from build123d import *

# Parameters (mm, degrees)
F0_R     = 42.5
F0_W     = 12
F0_H     = 12
F1_DEPTH = 15
F2_R     = 42.5
F3_DEPTH = 5
F4_R     = 2.1
F5_DEPTH = 10
F7_DEPTH = 4


with BuildPart() as f1:
    # F0 (on Top) → F1 (new body)
    with BuildSketch(Plane.XY):
        Circle(F0_R)
        Rectangle(F0_W, F0_H, mode=Mode.SUBTRACT)
    extrude(amount=F1_DEPTH)

    # F2 (on face) → F3 (join)
    with BuildSketch(Plane(origin=(0, 0, 0), x_dir=(1, 0, 0), z_dir=(0, 0, -1))):
        Circle(F2_R)
    extrude(amount=F3_DEPTH)

    # F4 (on face) → F5 (cut)
    with BuildSketch(Plane.XY.offset(15)):
        with Locations((-21.25, 0)):
            Circle(F4_R)
        with Locations((0, 21.25)):
            Circle(F4_R)
        with Locations((21.25, 0)):
            Circle(F4_R)
        with Locations((0, -21.25)):
            Circle(F4_R)
    extrude(amount=-F5_DEPTH, mode=Mode.SUBTRACT)

    # F6 (on face) → F7 (cut)
    with BuildSketch(Plane.XY.offset(15)):
        Polygon((-24.714102, 2), (-24.714102, -2), (-21.25, -4), (-17.785898, -2), (-17.785898, 2), (-21.25, 4), align=None)
        Polygon((-3.464102, 23.25), (-3.464102, 19.25), (0, 17.25), (3.464102, 19.25), (3.464102, 23.25), (0, 25.25), align=None)
        Polygon((17.785898, 2), (17.785898, -2), (21.25, -4), (24.714102, -2), (24.714102, 2), (21.25, 4), align=None)
        Polygon((-3.464102, -19.25), (-3.464102, -23.25), (0, -25.25), (3.464102, -23.25), (3.464102, -19.25), (0, -17.25), align=None)
    extrude(amount=-F7_DEPTH, mode=Mode.SUBTRACT)


solid = f1.part
Can you work these out from the model? Positions are in its coordinate system, mm. Coordinates: 2 decimals unless noted, no trailing zeros. Order: outer loops, then holes, each group sorted by start corner. A loop starts at its lowest first (then second) coordinate and runs counter-clockwise, first axis right, second up. Notation, with made-up numbers: M 85.25,20 L 140.25,20 A7 cw 140.25,25 Z; hole C 3,70 d7. An arc over 180 degrees is marked long. Answer as CSV lines item,"result".
(1) Suppose I cut it at C-C on z = -2.25. Please give me the cut outline in (x, y).
Geometry check:
outline,"C 0,0 d85"
(2) If we mould it in two halves opening along Y, with no side actions, what happens to faces 1 (the flat face through (-1.756, -24.236, 13.028)), 2 (the flat face through (-1, -1, -5))? For each: released by +Y, released by -Y, zero draft, split by the parting line, or undercut.
Geometry check:
face 1,"undercut"
face 2,"zero draft"
(3) Suppose I cut it at A-A on z = 13.5. Count the separate pieces of the cut face and the enclosed holes in it, plus the area to 3 significant figures.
Geometry check:
separate pieces,"1"
enclosed holes,"5"
area,"5,360 mm^2"
(4) Suppose I cut it at B-B on y = 21.25. Please give me the cut outline in (x, z).
Geometry check:
outline,"M -36.81,-5 L 36.81,-5 L 36.81,15 L 3.46,15 L 3.46,11 L 2.1,11 L 2.1,5 L -2.1,5 L -2.1,11 L -3.46,11 L -3.46,15 L -36.81,15 Z"
(5) Suppose I cut it at D-D on x = -34. Please give me the cut outline in (y, z), plus the area to 3 significant figures.
Geometry check:
outline,"M -25.5,-5 L 25.5,-5 L 25.5,15 L -25.5,15 Z"
area,"1,020 mm^2"
(6) I'm going to push flat-ended pins straight in: pin 1 (2 mm diameter, centred on y = 0.5, z = 12, fed in from -X); pin 2 (3.5 mm diameter, centred on x = -0.5, y = -20.5, fed in from +Z); pin 3 (1.5 mm diameter, centred on x = 27, z = 9.5, fed in from +Y); pin 4 (1.2 mm diameter, centred on y = 21.5, z = 12.5, fed in from -X). Where does each tip first touch, or does it pass through?
Geometry check:
pin 1,"x = -42.5"
pin 2,"z = 11"
pin 3,"y = 33.42"
pin 4,"x = -37.01"
(7) Please list where these lines run through material, in increasing order: L1, parallel to Y at x = 0, z = 9.65; L2, parallel to Y at x = -21.25, z = 6.55; L3, parallel to Y at x = -4.5, z = 2.75.
Geometry check:
L1,"-42.5 to -23.35, -19.15 to -6, 6 to 19.15, 23.35 to 42.5"
L2,"-36.81 to -2.1, 2.1 to 36.81"
L3,"-42.26 to -6, 6 to 42.26"
